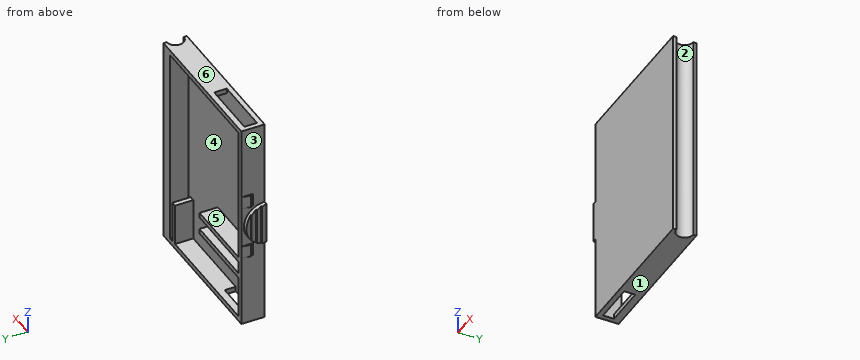
from build123d import *

# Parameters (mm, degrees)
SKETCH2_W            = 42
SKETCH2_H            = 64
BOSS_EXTRUDE1_DEPTH  = 1.6
SKETCH4_W            = 47.6
SKETCH4_H            = 67.2
SKETCH4_W_2          = 42
SKETCH4_H_2          = 64
BOSS_EXTRUDE2_DEPTH  = 6.6
BOSS_EXTRUDE3_DEPTH  = 1.6
CUT_EXTRUDE2_DEPTH   = 53.6
SKETCH12_W           = 18.5
SKETCH12_H           = 4
CUT_EXTRUDE5_DEPTH   = 4.5
SKETCH14_W           = 24
SKETCH14_H           = 7.2
BOSS_EXTRUDE6_DEPTH  = 5
SKETCH21_W           = 47.6
SKETCH21_H           = 67.2
BOSS_EXTRUDE8_DEPTH  = 0.8
SKETCH22_W           = 13
SKETCH22_H           = 3.5
CUT_EXTRUDE6_DEPTH   = 10.8
SKETCH26_W           = 24
SKETCH26_H           = 4
CUT_EXTRUDE7_DEPTH   = 5.8
SKETCH27_W           = 3
SKETCH27_H           = 13.4
BOSS_EXTRUDE9_DEPTH  = 5.8
SKETCH28_R           = 2.7
CUT_EXTRUDE8_DEPTH   = 70.8
SKETCH29_W           = 4
SKETCH29_H           = 3.7
BOSS_EXTRUDE10_DEPTH = 0.5
CUT_EXTRUDE9_DEPTH   = 4.5
CUT_EXTRUDE10_DEPTH  = 4.5
SKETCH38_W           = 1.4
SKETCH38_H           = 13.4
CUT_EXTRUDE12_DEPTH  = 5.8


with BuildPart() as part:
    # Sketch2 → Boss-Extrude1 (new body)
    with BuildSketch(Plane(origin=(0, 0, 0), x_dir=(1, 0, 0), z_dir=(0, 1, 0))):
        with Locations((21, -32)):
            Rectangle(SKETCH2_W, SKETCH2_H)
    extrude(amount=BOSS_EXTRUDE1_DEPTH)

    # Sketch4 → Boss-Extrude2 (add)
    with BuildSketch(Plane(origin=(0, 0, 0), x_dir=(1, 0, 0), z_dir=(0, 1, 0))):
        with Locations((22.2, -32)):
            Rectangle(SKETCH4_W, SKETCH4_H)
        with Locations((21, -32)):
            Rectangle(SKETCH4_W_2, SKETCH4_H_2, mode=Mode.SUBTRACT)
    extrude(amount=BOSS_EXTRUDE2_DEPTH)

    # Sketch6 → Boss-Extrude3 (add)
    with BuildSketch(Plane.ZY.offset(1.6)):
        with BuildLine():
            Line((25.4, 0), (38.6, 0))
            ThreePointArc((38.6, 0), (32, 6.6), (25.4, 0))
        make_face()
    extrude(amount=BOSS_EXTRUDE3_DEPTH)

    # Sketch7 → Cut-Extrude2 (cut)
    with BuildSketch(Plane.XY):
        Polygon((-3.2, 6.6), (-3.2, 4.95), (-2.7, 4.95), align=None)
        Polygon((-3.2, 4.95), (-3.2, 3.3), (-2.7, 3.3), align=None)
        Polygon((-2.7, 1.65), (-3.2, 3.3), (-3.2, 1.65), align=None)
        Polygon((-2.7, 0), (-3.2, 1.65), (-3.2, 0), align=None)
    extrude(amount=CUT_EXTRUDE2_DEPTH, mode=Mode.SUBTRACT)

    # Sketch12 → Cut-Extrude5 (cut)
    with BuildSketch(Plane(origin=(0, 0, 64), x_dir=(-1, 0, 0), z_dir=(0, 0, -1))):
        with Locations((-9.25, 3.6)):
            Rectangle(SKETCH12_W, SKETCH12_H)
    extrude(amount=-CUT_EXTRUDE5_DEPTH, mode=Mode.SUBTRACT)

    # Sketch14 → Boss-Extrude6 (add)
    with BuildSketch(Plane(origin=(0, 1.6, 0), x_dir=(1, 0, 0), z_dir=(0, 1, 0))):
        with Locations((12, -17)):
            Rectangle(SKETCH14_W, SKETCH14_H)
    extrude(amount=BOSS_EXTRUDE6_DEPTH)

    # Sketch21 → Boss-Extrude8 (add)
    with BuildSketch(Plane(origin=(0, 6.6, 0), x_dir=(1, 0, 0), z_dir=(0, 1, 0))):
        with Locations((22.2, -32)):
            Rectangle(SKETCH21_W, SKETCH21_H)
        Polygon((0, -13.4), (0, 0), (42, 0), (42, -64), (0, -64), (0, -20.6), (24, -20.6), (24, -13.4), align=None, mode=Mode.SUBTRACT)
    extrude(amount=BOSS_EXTRUDE8_DEPTH)

    # Sketch22 → Cut-Extrude6 (cut)
    with BuildSketch(Plane.XY):
        with Locations((6.5, 3.35)):
            Rectangle(SKETCH22_W, SKETCH22_H)
    extrude(amount=-CUT_EXTRUDE6_DEPTH, mode=Mode.SUBTRACT)

    # Sketch26 → Cut-Extrude7 (cut)
    with BuildSketch(Plane(origin=(0, 7.4, 0), x_dir=(1, 0, 0), z_dir=(0, 1, 0))):
        with Locations((12, -17)):
            Rectangle(SKETCH26_W, SKETCH26_H)
    extrude(amount=-CUT_EXTRUDE7_DEPTH, mode=Mode.SUBTRACT)

    # Sketch27 → Boss-Extrude9 (add)
    with BuildSketch(Plane(origin=(0, 1.6, 0), x_dir=(1, 0, 0), z_dir=(0, 1, 0))):
        with Locations((40.5, -6.7)):
            Rectangle(SKETCH27_W, SKETCH27_H)
    extrude(amount=BOSS_EXTRUDE9_DEPTH)

    # Sketch28 → Cut-Extrude8 (cut)
    with BuildSketch(Plane.XY.offset(65.6)):
        with Locations((46, 3.7)):
            Circle(SKETCH28_R)
    extrude(amount=-CUT_EXTRUDE8_DEPTH, mode=Mode.SUBTRACT)

    # Sketch29 → Boss-Extrude10 (add)
    with BuildSketch(Plane.ZY.offset(1.6)):
        with Locations((23.4, 5.55)):
            Rectangle(SKETCH29_W, SKETCH29_H)
        with Locations((40.6, 5.55)):
            Rectangle(SKETCH29_W, SKETCH29_H)
    extrude(amount=BOSS_EXTRUDE10_DEPTH)

    # Sketch30 → Cut-Extrude9 (cut)
    with BuildSketch(Plane(origin=(0, 0, 21.4), x_dir=(-1, 0, 0), z_dir=(0, 0, -1))):
        Polygon((2.1, 4.625), (2.1, 5.55), (2.1, 7.4), (1.6, 7.4), align=None)
        Polygon((2.1, 3.7), (2.1, 4.625), (1.6, 3.7), align=None)
    extrude(amount=-CUT_EXTRUDE9_DEPTH, mode=Mode.SUBTRACT)

    # Sketch31 → Cut-Extrude10 (cut)
    with BuildSketch(Plane.XY.offset(42.6)):
        Polygon((-2.1, 5.55), (-2.1, 4.625), (-1.6, 7.4), (-2.1, 7.4), align=None)
        Polygon((-2.1, 4.625), (-2.1, 3.7), (-1.6, 3.7), align=None)
    extrude(amount=-CUT_EXTRUDE10_DEPTH, mode=Mode.SUBTRACT)

    # Sketch38 → Cut-Extrude12 (cut)
    with BuildSketch(Plane(origin=(0, 7.4, 0), x_dir=(1, 0, 0), z_dir=(0, 1, 0))):
        with Locations((41.3, -6.7)):
            Rectangle(SKETCH38_W, SKETCH38_H)
    extrude(amount=-CUT_EXTRUDE12_DEPTH, mode=Mode.SUBTRACT)


solid = part.part
Read the model definition and answer for the solid it produces. Units are mm, in the model's axes. Face numbers are marked on the shaded views. A direction names the side the tool comes from. Coordinates: 2 decimals unless noted, no trailing zeros. Order: outer loops, then holes, each group sorted by start corner. A loop starts at its lowest first (then second) coordinate and runs counter-clockwise, first axis right, second up. Notation, with made-up numbers: (-29, -21) -> (0, -21) arc R22 cw to (0, -8) -> close; hole circle Ø9 at (-19, 64). An arc over 180 degrees is marked (long way). Answer as a JSON object with one key per item and string values.
1) A cutting plane is placed at A-A, the plane x = 16. Determine the outline of the cut face in (y, z), plus the area to 3 significant figures.
Model answer:
{"outline": "(0, -1.6) -> (7.4, -1.6) -> (7.4, 0) -> (1.6, 0) -> (1.6, 13.4) -> (7.4, 13.4) -> (7.4, 15) -> (1.6, 15) -> (1.6, 19) -> (7.4, 19) -> (7.4, 20.6) -> (1.6, 20.6) -> (1.6, 65.6) -> (0, 65.6) -> close; (5.6, 64) -> (7.4, 64) -> (7.4, 65.6) -> (5.6, 65.6) -> close", "area": "138 mm²"}
2) A cutting plane is placed at C-C, the plane z = 55. Determine the outline of the cut face in (x, y), plus the area to 3 significant figures.
Model answer:
{"outline": "(-1.6, 0) -> (46, 0) -> (46, 1) arc R2.7 cw to (46, 6.4) -> (46, 7.4) -> (42, 7.4) -> (42, 1.6) -> (0, 1.6) -> (0, 7.4) -> (-1.6, 7.4) -> close", "area": "97.2 mm²"}
3) The mould has two halves that part along X. Classify the marked faces 1, 2, 3 and 4: released by +X, released by -X, zero draft, split by the parting line, or undercut.
Model answer:
{"face 1": "zero draft", "face 2": "released by +X", "face 3": "released by -X", "face 4": "undercut"}
4) A cutting plane is placed at D-D, the plane z = 32. Determine the outline of the cut face in (x, y).
Model answer:
{"outline": "(-3.2, 1.65) -> (-2.7, 0) -> (46, 0) -> (46, 1) arc R2.7 cw to (46, 6.4) -> (46, 7.4) -> (42, 7.4) -> (42, 1.6) -> (0, 1.6) -> (0, 7.4) -> (-1.6, 7.4) -> (-1.6, 6.6) -> (-3.2, 6.6) -> (-2.7, 4.95) -> (-3.2, 4.95) -> (-2.7, 3.3) -> (-3.2, 3.3) -> (-2.7, 1.65) -> close"}
5) A tool of negligible diameter and unlimited length cuts with its end or side. For the marked faces 5 and 6, from which of +Z, -Z, +X, -X, +Y, -Y can it reach the whole face along a straight path? Write none if from no direction.
Model answer:
{"face 5": "+Y", "face 6": "+Z, +X, -X, +Y, -Y"}
6) A cutting plane is placed at B-B, the plane x = 3. Determine the outline of the cut face in (y, z).
Model answer:
{"outline": "(0, -1.6) -> (1.6, -1.6) -> (1.6, 13.4) -> (7.4, 13.4) -> (7.4, 15) -> (1.6, 15) -> (1.6, 19) -> (7.4, 19) -> (7.4, 20.6) -> (1.6, 20.6) -> (1.6, 65.6) -> (0, 65.6) -> close; (5.1, -1.6) -> (7.4, -1.6) -> (7.4, 0) -> (5.1, 0) -> close; (5.6, 64) -> (7.4, 64) -> (7.4, 65.6) -> (5.6, 65.6) -> close"}
7) Each of these flat-tipped pins is pushed along its axis until it touches: pin 1 (12 mm diameter, centred on x = 13.5, z = 39, fed in from +Y); pin 2 (3 mm diameter, centred on y = 4.5, z = 17, fed in from +X); pin 3 (0.8 mm diameter, centred on y = 5, z = 19.5, fed in from +X). Where does it stop, or does it pass through?
Model answer:
{"pin 1": "stops at y = 1.6", "pin 2": "stops at x = 44.59", "pin 3": "stops at x = 43.9"}
8) Consider line 1 along X through (y, z) = (4, 59); line 2 along X through (y, z) = (7.25, 18.5); line 3 along Z through (x, y) = (38, 6.5). Determine where each line is inside the solid, lowest interval first. Write a range as from..to.
Model answer:
{"line 1": "x = -1.6..0, 42..43.32", "line 2": "x = -1.6..0, 42..46", "line 3": "z = -1.6..0, 64..65.6"}
